Read the model definition and answer for the solid it produces. Units are mm, in the model's axes. A direction names the side the tool comes from. Coordinates: 2 decimals unless noted, no trailing zeros. Order: outer loops, then holes, each group sorted by start corner. A loop starts at its lowest first (then second) coordinate and runs counter-clockwise, first axis right, second up. Notation, with made-up numbers: (9, 35.25) - (37, 35.25) arc R11 cw to (37, 55.25) - close; hole circle Ø10 at (76, 10). An arc over 180 degrees is marked (long way). Answer as a JSON object with one key per item and string values. Group by question number.
from build123d import *

# Parameters (mm, degrees)
F1_DEPTH = 63.5
F2_DEPTH = 25.4
F3_DEPTH = 7.9375
F4_R     = 5.08


with BuildPart() as f1:
    # F0 (on Front) → F1 (new body, symmetric)
    with BuildSketch(Plane.XZ):
        Polygon((-41.275, 9.525), (-41.275, -9.525), (41.275, -9.525), (41.275, 9.525), (22.225, 9.525), align=None)
    extrude(amount=F1_DEPTH, both=True)

    # F0 (on Front) → F2 (join, symmetric)
    with BuildSketch(Plane.XZ):
        with BuildLine():
            Line((22.225, 9.525), (41.275, 9.525))
            Line((41.275, 9.525), (41.275, 27.0002))
            ThreePointArc((41.275, 27.0002), (45.92468, 38.22552), (57.15, 42.8752))
            Line((57.15, 42.8752), (60.325, 42.8752))
            Line((60.325, 42.8752), (60.325, 61.9252))
            Line((60.325, 61.9252), (57.15, 61.9252))
            add(Edge.make_bspline(
                [(56.444235, 61.918068), (56.679218, 61.920897), (56.914473, 61.923274), (57.15, 61.9252)],
                knots=[111.045003, 111.045003, 111.045003, 111.045003, 111.504536, 111.504536, 111.504536, 111.504536], degree=3))
            ThreePointArc((56.444235, 61.918068), (32.206018, 51.445105), (22.225, 27.0002))
            Line((22.225, 27.0002), (22.225, 9.525))
        make_face()
        Polygon((60.325, 66.675), (60.325, 61.9252), (60.325, 42.8752), (60.325, 38.1), (85.725, 38.1), (85.086263, 66.675), align=None)
    extrude(amount=F2_DEPTH, both=True)

    # F0 (on Front) → F3 (join, symmetric)
    with BuildSketch(Plane.XZ):
        with BuildLine():
            add(Edge.make_bspline(
                [(-41.275, 9.525), (-41.190063, 34.252091), (-0.338804, 61.234613), (56.444235, 61.918068)],
                knots=[0, 0, 0, 0, 111.045003, 111.045003, 111.045003, 111.045003], degree=3))
            Line((-41.275, 9.525), (22.225, 9.525))
            Line((22.225, 9.525), (22.225, 27.0002))
            ThreePointArc((22.225, 27.0002), (32.206018, 51.445105), (56.444235, 61.918068))
        make_face()
    extrude(amount=F3_DEPTH, both=True)

    # F4
    f4_edges = [f1.edges().sort_by_distance(p)[0] for p in [
        (41.275, -63.5, 0),
        (-41.275, -63.5, 0),
        (41.275, 63.5, 0),
        (-41.275, 63.5, 0),
    ]]
    fillet(f4_edges, radius=F4_R)


solid = f1.part
1. Given pin 1 (8 mm diameter, centred on x = 8, z = 23, fed in from -Y); pin 2 (19 mm diameter, centred on y = -17.5, z = 17, fed in from -X) (3 decimals); pin 3 (2 mm diameter, centred on x = 2.5, z = 35.5, fed in from +Y); pin 4 (1 mm diameter, centred on x = 59.5, y = 8.5, fed in from -Z), each flat-ended and moving along its own axis, determine where each tip first touches the part or whether it passes through.
2. A cutting plane is placed at A-A on z = -1. Write down the section's boundary in (x, y) (3 decimals).
3. A cutting plane is placed at C-C on x = 77. Write down the section's boundary in (y, z) (3 decimals), and give its area (3 significant figures).
4. A cutting plane is placed at B-B on y = 52. Write down the section's boundary in (x, z) (3 decimals).
5. For faces 4 (the flat face through (54, -25.4, 45)), 5 (the flat face through (73, 0, 38.1)), 6 (the flat face through (73, 0, 66.675)), 7 (the cylindrical face through (32.47, 16.55, 51.71)), 8 (the cylindrical face through (32.47, -16.79, 51.71)), determine the directions among +Z, -Z, +X, -X, +Y, -Y from which every point of the face is accessible in a straight line to the end or side of a thin tool.
6. Straight lines are drawn through the part: L1, parallel to X at y = -16.5, z = 24.5 (3 decimals); L2, parallel to Y at x = 22, z = 25; L3, parallel to Z at x = -16, y = -53 (3 decimals). For each, find the intervals that lie inside material, in ascending order.
7. For a pull along X with two mould halves and no side action, classify faces 1 (the flat face through (59, 0, 42.875)), 2 (the flat face through (60.325, 0, 64)), 3 (the flat face through (54, 25.4, 45)) as pulls with the +X half, pulls with the -X half, needs draft (parallel to the pull), parting line crosses it, or undercut.
Derived:
{
 "1": {"pin 1": "stops at y = -7.94", "pin 2": "stops at x = -41.275", "pin 3": "stops at y = 7.94", "pin 4": "stops at z = 42.88"},
 "2": {"outline": "(-41.275, -58.42) arc R5.08 ccw to (-36.195, -63.5) - (36.195, -63.5) arc R5.08 ccw to (41.275, -58.42) - (41.275, 58.42) arc R5.08 ccw to (36.195, 63.5) - (-36.195, 63.5) arc R5.08 ccw to (-41.275, 58.42) - close"},
 "3": {"outline": "(-25.4, 38.1) - (25.4, 38.1) - (25.4, 66.675) - (-25.4, 66.675) - close", "area": "1,450 mm2"},
 "4": {"outline": "(-41.275, -9.525) - (41.275, -9.525) - (41.275, 9.525) - (-41.275, 9.525) - close"},
 "5": {"face 4": "+Z, +X, -X, -Y", "face 5": "-Z, +X, +Y, -Y", "face 6": "+Z, +X, -X, +Y, -Y", "face 7": "+Z, -X, +Y", "face 8": "+Z, -X, -Y"},
 "6": {"L1": "x = 22.225 to 41.275", "L2": "y = -7.94 to 7.94", "L3": "z = -9.525 to 9.525"},
 "7": {"face 1": "undercut", "face 2": "pulls with the -X half", "face 3": "needs draft"}
}
